from build123d import *

# Parameters (mm, degrees)
F0_R     = 12.5
F1_DEPTH = 3


with BuildPart() as f1:
    # F0 (on Top) → F1 (new body)
    with BuildSketch(Plane.XY):
        with BuildLine():
            Line((-14, -4), (-17.036725, -4))
            ThreePointArc((-17.036725, -4), (0, -17.5), (17.036725, -4))
            Line((17.036725, -4), (14, -4))
            Line((14, -4), (14, 4))
            Line((14, 4), (17.036725, 4))
            ThreePointArc((17.036725, 4), (0, 17.5), (-17.036725, 4))
            Line((-17.036725, 4), (-14, 4))
            Line((-14, 4), (-14, -4))
        make_face()
        Circle(F0_R, mode=Mode.SUBTRACT)
    extrude(amount=F1_DEPTH)


solid = f1.part
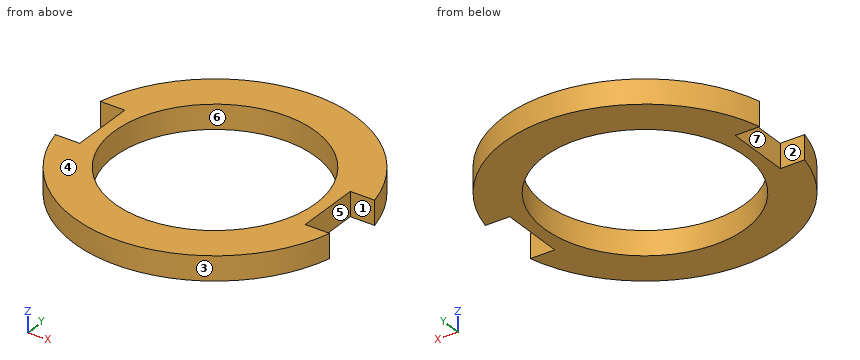
Can you work these out from the model? Positions are in its coordinate system, mm. Face numbers are marked on the shaded views. A direction names the side the tool comes from. Coordinates: 2 decimals unless noted, no trailing zeros. Order: outer loops, then holes, each group sorted by start corner. A loop starts at its lowest first (then second) coordinate and runs counter-clockwise, first axis right, second up. Notation, with made-up numbers: M 2,81 L 56,81 A13 ccw 56,90 Z; hole C 23.5,5 d7. An arc over 180 degrees is marked long. Answer as CSV lines item,"result".
(1) Suppose I cut it at B-B on z = 1.35. Please give me the cut outline in (x, y).
Geometry check:
outline,"M -17.04,-4 A17.5 ccw 17.04,-4 L 14,-4 L 14,4 L 17.04,4 A17.5 ccw -17.04,4 L -14,4 L -14,-4 Z; hole C 0,0 d25"
(2) On a 3-axis mill with a long thin cutter (end or side, diameter ignored), from which of +Z, -Z, +X, -X, +Y, -Y can I reach the whole of each face in a straight line? I mean the marked faces 1, 2 and 3. Say none if no direction works.
Geometry check:
face 1,"+Z, -Z, +X"
face 2,"+Z, -Z, -X"
face 3,"+Z, -Z, -Y"
(3) Suppose I cut it at D-D on y = 14. Please give me the cut outline in (x, z), plus the area to 3 significant figures.
Geometry check:
outline,"M -10.5,0 L 10.5,0 L 10.5,3 L -10.5,3 Z"
area,"63.0 mm^2"
(4) Suppose I cut it at C-C on y = 0. Please give me the cut outline in (x, z).
Geometry check:
outline,"M -14,0 L -12.5,0 L -12.5,3 L -14,3 Z; M 12.5,0 L 14,0 L 14,3 L 12.5,3 Z"
(5) Please list where these lines run through material, in increasing order: L1, parallel to Y at x = 3.5, z = 1.9; L2, parallel to X at y = -9.5, z = 1.7; L3, parallel to Y at x = 7, z = 2.15.
Geometry check:
L1,"-17.15 to -12, 12 to 17.15"
L2,"-14.7 to -8.12, 8.12 to 14.7"
L3,"-16.04 to -10.36, 10.36 to 16.04"
(6) I'm going to push flat-ended pins straight in: pin 1 (1.5 mm diameter, centred on x = 15, z = 1, fed in from -Y); pin 2 (1.5 mm diameter, centred on x = -15.5, z = 1.5, fed in from -Y); pin 3 (0.9 mm diameter, centred on y = -0.5, z = 1, fed in from -X). Where does each tip first touch, or does it pass through?
Geometry check:
pin 1,"y = -10.16"
pin 2,"y = -9.42"
pin 3,"x = -14"
(7) Suppose I cut it at A-A on x = 0. Please give me the cut outline in (y, z).
Geometry check:
outline,"M -17.5,0 L -12.5,0 L -12.5,3 L -17.5,3 Z; M 12.5,0 L 17.5,0 L 17.5,3 L 12.5,3 Z"
(8) If we mould it in two halves opening along X, with no side actions, what happens to the marked faces 4, 5, 6 and 7? For each: released by +X, released by -X, zero draft, split by the parting line, or undercut.
Geometry check:
face 4,"zero draft"
face 5,"released by +X"
face 6,"undercut"
face 7,"released by -X"
